Autodesk Inventor part; units mm, degrees
ref_plane "YZ Plane" through (0, 0, 0) normal (1, 0, 0) x (0, 1, 0)
ref_plane "XZ Plane" through (0, 0, 0) normal (0, 1, 0) x (-1, 0, 0)
ref_plane "XY Plane" through (0, 0, 0) normal (0, 0, 1) x (1, 0, 0)
sketch "Sketch1" plane through (0, 0, 0) normal (0, 0, 1) x (1, 0, 0)
  line L0 (-10.5, 6) -> (10.5, 6)
  line L1 (10.5, 6) -> (10.5, -6)
  line L2 (10.5, -6) -> (-10.5, -6)
  line L3 (-10.5, -6) -> (-10.5, 6)
  line L4 (-10.5, 6) -> (10.5, -6) construction
  line L5 (10.5, 6) -> (-10.5, -6) construction
  point P0 (0, 0)
  dimension "d0" = 21
  dimension "d1" = 12
extrude "Extrusion1" add sketch "Sketch1" along normal blind 9
chamfer "Chamfer1" distance 0.5 angle 45 12 edges at (0, 6, 9) (-10.5, 0, 9) (10.5, 0, 9) (0, -6, 9) (10.5, 6, 4.5) (10.5, -6, 4.5) (10.5, 0, 0) (-10.5, 6, 4.5) (-10.5, -6, 4.5) (0, -6, 0) (-10.5, 0, 0) (0, 6, 0)
sketch "Sketch2" plane through (0, 0, 9) normal (0, 0, 1) x (1, 0, 0)
  circle A0 centre (4, 0) radius 4.25
  line L0 (10.5, -5.5) -> (10.5, 5.5)
  point P0 (0, 0)
  dimension "d7" = 8.5
  dimension "d8" = 6.5
extrude "Extrusion2" cut sketch "Sketch2" against normal through all
sketch "Sketch3" plane through (-10, 6, 0.5) normal (0, 1, 0) x (1, 0, 0)
  line L0 (20, 0) -> (20, -8)
  circle A0 centre (13.5, -4) radius 1
  point P0 (10, 0.5)
  point P1 (20, -4)
  point P2 (20, -4)
  dimension "d11" = 2
  dimension "d12" = 6.5
extrude "Extrusion3" cut sketch "Sketch3" against normal up to surface
sketch "Sketch4" plane through (-10.5, -5.5, 0.5) normal (-1, 0, 0) x (0, 0, 1)
  point P0 (-0.5, 5.5)
  point P1 (4, 5.5)
hole "Hole1" at (-10.5, 0, 4.5) direction (1, 0, 0) diameter 4.917 depth 10
properties part number "16B2 - Con Head Big End" material "Steel AISI 1020 107 HR"
Geometry: final body of the model. Coordinates: model frame, mm. A direction names the side the tool comes from. Give positions to 0.01 mm unless a question says otherwise; leave off trailing zeros. Loops run counter-clockwise (first coordinate to the right, second up) from the corner with the lowest first, then second, coordinate; pieces in that order, holes last. Notation, with made-up numbers: M 56,15.25 L 65,15.25 A31 cw 65,43.25 Z; hole C 40.5,-16 d5. An arc over 180 degrees is marked long. Put each result on its own line as item: value.
1) Cut plane A-A, the plane y = 5.25. Return the cut outline in (x, z), plus the area to 3 significant figures.
Computed values:
outline: M -10.5,0.5 L -10,0 L 10,0 L 10.5,0.5 L 10.5,8.5 L 10,9 L -10,9 L -10.5,8.5 Z; hole C 3.5,4.5 d2
area: 185 mm^2
2) Material intervals for L1, parallel to Y at x = -5, z = 4.5; L2, parallel to Z at x = -7.5, y = 0; L3, parallel to Y at x = 4, z = 2.75, sorted ascending. Write a range as from..to.
Computed values:
L1: y = -6..-2.46, 2.46..6
L2: z = 0..2.04, 6.96..9
L3: y = -6..-4.25, 4.25..6
3) Cut plane B-B, the plane x = -7. Return the cut outline in (y, z).
Computed values:
outline: M -6,0.5 L -5.5,0 L 5.5,0 L 6,0.5 L 6,8.5 L 5.5,9 L -5.5,9 L -6,8.5 Z; hole C 0,4.5 d4.92
4) First-contact query: P1, Ø5, axis at x = 4, y = 0, coming from the -Z side. Flat tip, straight axial feed; report the tip coordinate or a pass-through.
Computed values:
P1: passes through
5) Cut plane D-D, the plane x = 7.75. Return the cut outline in (y, z), plus the area to 3 significant figures.
Computed values:
outline: M -6,0.5 L -5.5,0 L -2,0 L -2,9 L -5.5,9 L -6,8.5 Z; M 2,0 L 5.5,0 L 6,0.5 L 6,8.5 L 5.5,9 L 2,9 Z
area: 71.5 mm^2
6) Reachability of faces 5 (the cylindrical face through (-5.43, -0.108, 2.044)), 6 (the flat face through (-10.5, -3, 4)) from +Z, -Z, +X, -X, +Y, -Y: full face, straight path, thin tool, end or side. Return the list, or none.
Computed values:
face 5: -X
face 6: +Z, -Z, -X, +Y, -Y
7) Mould query, pull axis X, two halves, no side actions, for faces 1 (the flat face through (10.5, 0, 4)), 2 (the cylindrical face through (3.08, -4.15, 4.56)), 3 (the cylindrical face through (2.5, 5, 4.5)), 4 (the flat face through (-2, 0, 9)). Classes: released by +X, released by -X, zero draft, split by the parting line, or undercut.
Computed values:
face 1: released by +X
face 2: undercut
face 3: undercut
face 4: zero draft
8) Cut plane C-C, the plane y = 0. Return the cut outline in (x, z).
Computed values:
outline: M -10.5,0.5 L -10,0 L -0.25,0 L -0.25,9 L -10,9 L -10.5,8.5 L -10.5,6.96 L -0.5,6.96 L -0.5,2.04 L -10.5,2.04 Z; M 8.25,0 L 10,0 L 10.5,0.5 L 10.5,8.5 L 10,9 L 8.25,9 Z
